Could you check a few things on this model? Use its own coordinates, in mm. A direction names the side the tool comes from. Round coordinates to 2 decimals unless told otherwise and drop trailing zeros. Loops run counter-clockwise (first coordinate to the right, second up) from the corner with the lowest first, then second, coordinate; pieces in that order, holes last. Notation, with made-up numbers: M -26,-20.75 L -1,-20.75 A23 ccw -1,-7.75 Z; hole C -12.75,73 d5. An arc over 180 degrees is marked long. Answer in a Markdown table with one row per item.
```python
from build123d import *

# Parameters (mm, degrees)
F0_W     = 75
F0_H     = 50
F1_DEPTH = 25
F2_W     = 5
F2_H     = 7.5
F3_DEPTH = 1.5
F4_R     = 2.5
F5_DEPTH = 15


with BuildPart() as f1:
    # F0 (on Top) → F1 (new body)
    with BuildSketch(Plane.XY):
        Rectangle(F0_W, F0_H)
    extrude(amount=F1_DEPTH)

    # F2 (on face) → F3 (cut)
    with BuildSketch(Plane.XY.offset(25)):
        with BuildLine():
            Line((-21.5, -12), (21.5, -12))
            ThreePointArc((21.5, -12), (24.328427, -10.828427), (25.5, -8))
            Line((25.5, -8), (25.5, 8))
            ThreePointArc((25.5, 8), (24.328427, 10.828427), (21.5, 12))
            Line((21.5, 12), (-21.5, 12))
            ThreePointArc((-21.5, 12), (-24.328427, 10.828427), (-25.5, 8))
            Line((-25.5, 8), (-25.5, -8))
            ThreePointArc((-25.5, -8), (-24.328427, -10.828427), (-21.5, -12))
        make_face()
        with Locations((-4, -5.25)):
            Rectangle(F2_W, F2_H, mode=Mode.SUBTRACT)
        with Locations((4, -5.25)):
            Rectangle(F2_W, F2_H, mode=Mode.SUBTRACT)
        with BuildLine():
            Line((-9.5, 9), (-9.5, -9))
            Line((-9.5, -9), (-21.5, -9))
            ThreePointArc((-21.5, -9), (-22.207107, -8.707107), (-22.5, -8))
            Line((-22.5, -8), (-22.5, 8))
            ThreePointArc((-22.5, 8), (-22.207107, 8.707107), (-21.5, 9))
            Line((-21.5, 9), (-9.5, 9))
        make_face(mode=Mode.SUBTRACT)
        with Locations((-4, 5.25)):
            Rectangle(F2_W, F2_H, mode=Mode.SUBTRACT)
        with Locations((4, 5.25)):
            Rectangle(F2_W, F2_H, mode=Mode.SUBTRACT)
        with BuildLine():
            ThreePointArc((22.5, -8), (22.207107, -8.707107), (21.5, -9))
            Line((21.5, -9), (9.5, -9))
            Line((9.5, -9), (9.5, 9))
            Line((9.5, 9), (21.5, 9))
            ThreePointArc((21.5, 9), (22.207107, 8.707107), (22.5, 8))
            Line((22.5, 8), (22.5, -8))
        make_face(mode=Mode.SUBTRACT)
    extrude(amount=-F3_DEPTH, mode=Mode.SUBTRACT)

    # F4 (on face) → F5 (cut)
    with BuildSketch(Plane.XY.offset(25)):
        Circle(F4_R)
    extrude(amount=-F5_DEPTH, mode=Mode.SUBTRACT)


solid = f1.part
```
1) Which directions (+Z, -Z, +X, -X, +Y, -Y) give clear straight access to the entire face, cutting with the end or side of a thin tool? Please do faces 1 (the face through (4, 9, 24)), 2 (the face through (-4, 5, 25)).
Computed:
| item | result |
|---|---|
| face 1 | +Z |
| face 2 | +Z, +X, -X, +Y, -Y |
2) I need wall thicknesses on line 1 (X direction, y = -7.5, z = 23.75); line 2 (X direction, y = 0, z = 21.25); line 3 (Y direction, x = 0, z = 13.5). Which ranges of each line are inside material? Lowest first, please.
Computed:
| item | result |
|---|---|
| line 1 | x = -37.5 to -25.5, -22.5 to -9.5, -6.5 to -1.5, 1.5 to 6.5, 9.5 to 22.5, 25.5 to 37.5 |
| line 2 | x = -37.5 to -2.5, 2.5 to 37.5 |
| line 3 | y = -25 to -2.5, 2.5 to 25 |
3) If we mould it in two halves opening along X, with no side actions, what happens to faces 3 (the face through (-6, 0, 23.5)), 4 (the face through (-1, 25, 12)), 5 (the face through (-37.5, 0, 12))? For each: released by +X, released by -X, zero draft, split by the parting line, or undercut.
Computed:
| item | result |
|---|---|
| face 3 | undercut |
| face 4 | zero draft |
| face 5 | released by -X |
4) I want a section at D-D, the plane y = -10. Please give me the cut outline in (x, z), plus the area to 3 significant figures.
Computed:
| item | result |
|---|---|
| outline | M -37.5,0 L 37.5,0 L 37.5,25 L 24.96,25 L 24.96,23.5 L -24.96,23.5 L -24.96,25 L -37.5,25 Z |
| area | 1,800 mm² |
5) I want a section at A-A, the plane y = 0. Please give me the cut outline in (x, z), plus the area to 3 significant figures.
Computed:
| item | result |
|---|---|
| outline | M -37.5,0 L 37.5,0 L 37.5,25 L 25.5,25 L 25.5,23.5 L 22.5,23.5 L 22.5,25 L 9.5,25 L 9.5,23.5 L 2.5,23.5 L 2.5,10 L -2.5,10 L -2.5,23.5 L -9.5,23.5 L -9.5,25 L -22.5,25 L -22.5,23.5 L -25.5,23.5 L -25.5,25 L -37.5,25 Z |
| area | 1,770 mm² |
6) I want a section at C-C, the plane x = 0. Please give me the cut outline in (y, z), plus the area to 3 significant figures.
Computed:
| item | result |
|---|---|
| outline | M -25,0 L 25,0 L 25,25 L 12,25 L 12,23.5 L 2.5,23.5 L 2.5,10 L -2.5,10 L -2.5,23.5 L -12,23.5 L -12,25 L -25,25 Z |
| area | 1,150 mm² |
7) I want a section at B-B, the plane x = 8.5. Please give me the cut outline in (y, z), plus the area to 3 significant figures.
Computed:
| item | result |
|---|---|
| outline | M -25,0 L 25,0 L 25,25 L 12,25 L 12,23.5 L -12,23.5 L -12,25 L -25,25 Z |
| area | 1,210 mm² |
8) Will this pin go through, and if not, where does the flat tip stop? P1, Ø1.5, axis at x = -1, y = 0, coming from the +Z side.
Computed:
| item | result |
|---|---|
| P1 | stops at z = 10 |
